For this review, take the finished solid that the model builds, in its own axes (mm). A direction names the side the tool comes from. Coordinates: 2 decimals unless noted, no trailing zeros. Loops run counter-clockwise (first coordinate to the right, second up) from the corner with the lowest first, then second, coordinate; pieces in that order, holes last.
Autodesk Inventor part; units mm, degrees
ref_plane "YZ Plane" through (0, 0, 0) normal (1, 0, 0) x (0, 1, 0)
ref_plane "XZ Plane" through (0, 0, 0) normal (0, 1, 0) x (-1, 0, 0)
ref_plane "XY Plane" through (0, 0, 0) normal (0, 0, 1) x (1, 0, 0)
sketch "Эскиз1" plane through (0, 0, 0) normal (0, 0, 1) x (1, 0, 0)
  line L0 (0, 0) -> (27.2, 0)
  line L1 (27.2, 0) -> (27.2, 22.4859)
  line L2 (12.2, 15) -> (0, 15)
  line L3 (0, 15) -> (0, 0)
  line L4 (27.2, 0) -> (21.9283, 0)
  line L5 (12.2, 15) -> (12.2, 70)
  line L6 (12.2, 70) -> (27.2, 70)
  line L7 (27.2, 70) -> (27.2, 0)
  line L8 (0, 0) -> (-35.2, 0)
  line L9 (-12.2, 15) -> (0, 15)
  line L10 (-20.2, 26.4) -> (-20.2, 55)
  line L11 (-20.2, 70) -> (-35.2, 70)
  line L12 (-35.2, 70) -> (-35.2, 0)
  line L13 (-12.2, 15) -> (-12.2, 26.4)
  line L14 (-12.2, 26.4) -> (-20.2, 26.4)
  line L15 (-20.2, 70) -> (-12.2, 70)
  line L16 (-12.2, 70) -> (-12.2, 55)
  line L17 (-12.2, 55) -> (-20.2, 55)
  line L18 (12.2, 60) -> (12.2, 70)
  dimension "d37" = 11.4
  dimension "d38" = 8
  dimension "d40" = 15
  dimension "d41" = 70
  dimension "d45" = 12.2
  dimension "d54" = 23
  dimension "d55" = 15
  dimension "d56" = 23
  dimension "d57" = 15
  dimension "d58" = 15
  dimension "d60" = 12.2
extrude "Выдавливание1" add sketch "Эскиз1" along normal blind 14 and the other way blind 5
sketch "Эскиз3" plane through (0, 0, -5) normal (0, 0, -1) x (-1, 0, 0)
  circle A0 centre (28.98, 17) radius 1.25
  circle A1 centre (3.98, 8.5) radius 1.25
  circle A2 centre (-21.02, 17) radius 1.25
  line L0 (-27.2, 0) -> (35.2, 0)
  circle A3 centre (29, 33.5) radius 1.25
  circle A4 centre (-21, 33.5) radius 1.25
  point P0 (0, 0)
  point P1 (4, 0)
  dimension "d10" = 2.5
  dimension "d12" = 8.5
  dimension "d14" = 50
  dimension "d27" = 17
  dimension "d28" = 25
  dimension "d29" = 17
  dimension "d30" = 25
extrude "Выдавливание3" cut sketch "Эскиз3" against normal up to surface (19 mm away)
fillet "Сопряжение1" radius 5 4 edges at (27.2, 0, 4.5) (-35.2, 70, 4.5) (12.2, 70, 4.5) (27.2, 70, 4.5)
sketch "Эскиз5" plane through (-35.2, 0, -5) normal (-1, 0, 0) x (0, -1, 0)
  circle A0 centre (-20.5, 11) radius 1.5
  circle A1 centre (-59.5, 11) radius 1.5
  point P0 (0, 5)
extrude "Выдавливание5" cut sketch "Эскиз5" against normal up to surface (23 mm away)
sketch "Эскиз6" plane through (27.2, 5, 14) normal (1, 0, 0) x (0, 0, -1)
  circle A0 centre (8, 15.5) radius 1.5
  circle A1 centre (8, 54.5) radius 1.5
  point P0 (14, -5)
extrude "Выдавливание6" cut sketch "Эскиз6" against normal up to surface (15 mm away)
sketch "Эскиз7" plane through (27.2, 5, 14) normal (1, 0, 0) x (0, 0, -1)
  circle A0 centre (8, 15.5) radius 3.5
  circle A1 centre (8, 54.5) radius 3.5
  circle A2 centre (8, 15.5) radius 1.5 construction
  circle A3 centre (8, 54.5) radius 1.5 construction
  point P0 (14, -5)
  dimension "d47" = 7
extrude "Выдавливание7" cut sketch "Эскиз7" against normal blind 4
sketch "Эскиз8" plane through (-35.2, 0, -5) normal (-1, 0, 0) x (0, 0, -1)
  circle A0 centre (-11, -20.5) radius 1.5 construction
  circle A1 centre (-11, -59.5) radius 1.5 construction
  line L0 (0, -15) -> (-19, -15)
  circle A2 centre (-11, -20.5) radius 3.5
  circle A3 centre (-11, -59.5) radius 3.5
  point P0 (-5, 0)
extrude "Выдавливание8" cut sketch "Эскиз8" against normal blind 4
fillet "Сопряжение2" radius 7 1 edges at (-35.2, 0, 4.5)
properties part number "Крепление стрелялки"
Q1. Consider section B-B (z = -2.5). State the section outline as (x, y) points, then the cut area to 3 significant figures.
Q2. For pin 1 Ø1.5 at (x, y) = (21, 33.5) entering from +Z; pin 2 Ø4 at (y, z) = (59.5, 6) entering from -X; pin 3 Ø5 at (y, z) = (59.5, 6) entering from +X, all flat-tipped, find the tip position at first contact; note any pin that passes through.
Q3. Consider section C-C (x = 21.02). State the section outline as (y, z) points, then the cut area to 3 significant figures.
Q4. Consider section D-D (y = 33.5). State the section outline as (x, z) points, then the cut area to 3 significant figures.
Q5. The part is to be moulded in two halves that separate along Y. For faces 1 (the face through (13.63, 68.5, 4.37)), 2 (the face through (-31.2, 59, 4)), 3 (the face through (12.2, 40, 4)), 4 (the face through (19.83, 17.38, 4.37)), say which applies: +Y half, -Y half, draft (parallel to the pull), parting line (faces both ways), or undercut.
Q6. Consider section A-A (y = 25). State the section outline as (x, z) points.
Q7. Wall thickness on probe 1 along Z at (x, y) = (-32.7, 59.5); probe 2 along Z at (x, y) = (-17.25, 20.5); probe 3 along X at (y, z) = (42, -3): over which ranges is each line inside the solid? List them lowest first.
Q8. Machinability: for faces 5 (the face through (-33, 17, 6)), 6 (the face through (-20.2, 40, 4)), 7 (the face through (23.2, 60, 4)), which of the approach directions +Z, -Z, +X, -X, +Y, -Y give a long, thin tool a straight path to every point of the face, cutting with its end or side? Answer none if there is none.
Model answer:
1. outline: (-35.2, 7) arc R7 ccw to (-28.2, 0) - (22.2, 0) arc R5 ccw to (27.2, 5) - (27.2, 65) arc R5 ccw to (22.2, 70) - (17.2, 70) arc R5 ccw to (12.2, 65) - (12.2, 15) - (-12.2, 15) - (-12.2, 26.4) - (-20.2, 26.4) - (-20.2, 55) - (-12.2, 55) - (-12.2, 70) - (-30.2, 70) arc R5 ccw to (-35.2, 65) - close; hole circle Ø2.5 at (-29, 33.5); hole circle Ø2.5 at (-28.98, 17); hole circle Ø2.5 at (-3.98, 8.5); hole circle Ø2.5 at (21, 33.5); hole circle Ø2.5 at (21.02, 17)
1. area: 2,740 mm2
2. pin 1: passes through
2. pin 2: stops at x = -31.2
2. pin 3: stops at x = 23.2
3. outline: (0, -5) - (15.75, -5) - (15.75, 14) - (0, 14) - close; (18.25, -5) - (32.25, -5) - (32.25, 14) - (18.25, 14) - close; (34.75, -5) - (70, -5) - (70, 14) - (34.75, 14) - close; hole circle Ø3 at (20.5, 6); hole circle Ø3 at (59.5, 6)
3. area: 1,220 mm2
4. outline: (-35.2, -5) - (-30.25, -5) - (-30.25, 14) - (-35.2, 14) - close; (-27.75, -5) - (-20.2, -5) - (-20.2, 14) - (-27.75, 14) - close; (12.2, -5) - (19.75, -5) - (19.75, 14) - (12.2, 14) - close; (22.25, -5) - (27.2, -5) - (27.2, 14) - (22.25, 14) - close
4. area: 475 mm2
5. face 1: +Y half
5. face 2: undercut
5. face 3: draft
5. face 4: undercut
6. outline: (-35.2, -5) - (-12.2, -5) - (-12.2, 14) - (-35.2, 14) - close; (12.2, -5) - (27.2, -5) - (27.2, 14) - (12.2, 14) - close
7. probe 1: z = -5 to 2.5, 9.5 to 14
7. probe 2: z = -5 to 4.5, 7.5 to 14
7. probe 3: x = -35.2 to -20.2, 12.2 to 27.2
8. face 5: -X
8. face 6: +Z, -Z
8. face 7: +X
